from build123d import *

# Parameters (mm, degrees)
BOSS_EXTRUDE1_DEPTH = 11.1125
CUT_EXTRUDE1_REACH  = 39.601
SKETCH4_R           = 3.5687
CUT_EXTRUDE2_DEPTH  = 38.600633818


with BuildPart() as part:
    # Sketch2 → Boss-Extrude1 (new, symmetric)
    with BuildSketch(Plane.XY):
        with BuildLine():
            Line((0, 0), (0, 25.4))
            Line((0, 25.4), (0.0127, 25.4))
            ThreePointArc((0.0127, 25.4), (3.380296045, 24.005096045), (4.7752, 20.6375))
            Line((4.7752, 20.6375), (4.7752, 7.9502))
            ThreePointArc((4.7752, 7.9502), (5.70513597, 5.70513597), (7.9502, 4.7752))
            Line((7.9502, 4.7752), (20.6375, 4.7752))
            ThreePointArc((20.6375, 4.7752), (24.005096045, 3.380296045), (25.4, 0.0127))
            Line((25.4, 0.0127), (25.4, 0))
            Line((25.4, 0), (0, 0))
        make_face()
    extrude(amount=BOSS_EXTRUDE1_DEPTH, both=True)

    # Sketch3 → Cut-Extrude1 (cut, up to next)
    with BuildSketch(Plane.ZY, mode=Mode.PRIVATE) as cut_extrude1_sk1:
        with BuildLine():
            Line((-3.5687, 17.4752), (-3.5687, 12.7))
            ThreePointArc((-3.5687, 12.7), (0, 9.1313), (3.5687, 12.7))
            Line((3.5687, 12.7), (3.5687, 17.4752))
            ThreePointArc((3.5687, 17.4752), (0, 21.0439), (-3.5687, 17.4752))
        make_face()
    cut_extrude1_tool1 = extrude(cut_extrude1_sk1.sketch, amount=-CUT_EXTRUDE1_REACH, mode=Mode.PRIVATE) & part.part
    add(cut_extrude1_tool1.solids().sort_by_distance((0, 15.0876, 0))[0], mode=Mode.SUBTRACT)

    # Sketch4 → Cut-Extrude2 (cut, through all)
    with BuildSketch(Plane.XZ):
        with Locations((12.7, 0)):
            Circle(SKETCH4_R)
    extrude(amount=-CUT_EXTRUDE2_DEPTH, mode=Mode.SUBTRACT)


solid = part.part
Build history of the part. All positions in model axes, mm. A direction names the side the tool comes from. Give positions to 0.01 mm unless a question says otherwise; leave off trailing zeros. Order: outer loops, then holes, each group sorted by start corner. A loop starts at its lowest first (then second) coordinate and runs counter-clockwise, first axis right, second up. Notation, with made-up numbers: M 48,34.5 L 65,34.5 A7 cw 65,39.5 Z; hole C 9,23.5 d3. An arc over 180 degrees is marked long. Use one line per item in the form item = value.
1) Drop flat-ended pins along their axis: pin 1 (1.5 mm diameter, centred on x = 7.5, y = 9, fed in from -Z); pin 2 (10 mm diameter, centred on x = 6, y = 14.5, fed in from -Z); pin 3 (4 mm diameter, centred on y = 15, z = 4.5, fed in from +X); pin 4 (8 mm diameter, centred on x = 12.7, z = 0, fed in from +Y). Give the stop position or say it passes through.
Calculated:
pin_1 = through
pin_2 = -11.11
pin_3 = 4.78
pin_4 = 4.78
2) Tool access for faces 1 (the face through (2, 15, 3.569)), 2 (the face through (0, 10, 3)), 3 (the face through (4.775, 10, 3)): list every direction of +Z, -Z, +X, -X, +Y, -Y with a clear straight run to the whole face (end or side of a thin tool).
Calculated:
face_1 = +X, -X
face_2 = +Z, -Z, -X, +Y, -Y
face_3 = +Z, -Z, +X, +Y
3) Two-plate mould, pull along Z, no slides. Class faces 4 (the face through (7, 4, -11.112)), 5 (the face through (23.968, 3.417, 0.156)), 6 (the face through (7, 4, 11.112)), 7 (the face through (2, 15, -3.569)): released by +Z, released by -Z, zero draft, split by the parting line, or undercut.
Calculated:
face_4 = released by -Z
face_5 = zero draft
face_6 = released by +Z
face_7 = undercut
4) Saw through at A-A (x = 12.7). Give the cut face in (y, z).
Calculated:
outline = M 0,-11.11 L 4.78,-11.11 L 4.78,-3.57 L 0,-3.57 Z; M 0,3.57 L 4.78,3.57 L 4.78,11.11 L 0,11.11 Z
5) Probe probe 1 along Z at (x, y) = (12.7, 1.9); probe 2 along Y at (x, z) = (15.5, -9.75); probe 3 along Y at (x, z) = (4, -3). List the from-to ranges inside material, lowest first.
Calculated:
probe_1 = -11.11 to -3.57, 3.57 to 11.11
probe_2 = 0 to 4.78
probe_3 = 0 to 10.77, 19.41 to 23.24
6) Saw through at C-C (y = 10.5). Give the cut face in (x, z), plus the area to 3 significant figures.
Calculated:
outline = M 0,-11.11 L 4.78,-11.11 L 4.78,-2.81 L 0,-2.81 Z; M 0,2.81 L 4.78,2.81 L 4.78,11.11 L 0,11.11 Z
area = 79.3 mm2
7) Saw through at B-B (z = -1.25). State how many separate pieces and enclosed holes the cut face has, plus the area to 3 significant figures.
Calculated:
separate_pieces = 3
enclosed_holes = 0
area = 126 mm2
